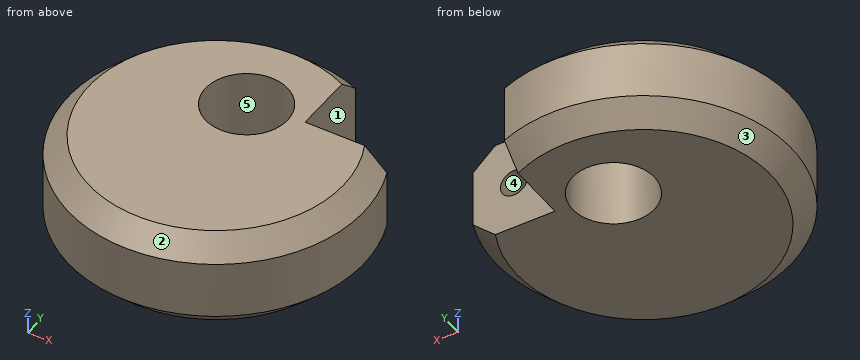
from build123d import *

# Parameters (mm, degrees)
SKETCH1_R             = 18
BOSS_EXTRUDE1_DEPTH   = 12
CUT_EXTRUDE4_DEPTH    = 17
SKETCH1_5_R           = 5
CUT_EXTRUDE5_DEPTH    = 22
M4_TAPPED_HOLE1_D     = 3.3
M4_TAPPED_HOLE1_DEPTH = 14
M4_TAPPED_HOLE1_TIP   = 0.991420021
CHAMFER1_SIZE         = 2.5
CHAMFER2_SIZE         = 2.5


with BuildPart() as part:
    # Sketch1 → Boss-Extrude1 (new body)
    with BuildSketch(Plane.XY):
        Circle(SKETCH1_R)
    extrude(amount=-BOSS_EXTRUDE1_DEPTH)

    # Sketch1<4> → Cut-Extrude4 (cut)
    with BuildSketch(Plane.XY):
        with BuildLine():
            Line((16.704699911, 6.704699911), (6.704699911, 6.704699911))
            Line((6.704699911, 6.704699911), (6.704699911, 16.704699911))
            ThreePointArc((6.704699911, 16.704699911), (12.727922061, 12.727922061), (16.704699911, 6.704699911))
        make_face()
    extrude(amount=-CUT_EXTRUDE4_DEPTH, mode=Mode.SUBTRACT)

    # Sketch1<5> → Cut-Extrude5 (cut)
    with BuildSketch(Plane.XY):
        with Locations((0, 6)):
            Circle(SKETCH1_5_R)
    extrude(amount=-CUT_EXTRUDE5_DEPTH, mode=Mode.SUBTRACT)

    # M4 Tapped Hole1
    with Locations(Plane(origin=(0, 6.704699911, 0), x_dir=(1, 0, 0), z_dir=(0, 1, 0))):
        with Locations((11.704699911, 6)):
            Hole(M4_TAPPED_HOLE1_D / 2, depth=M4_TAPPED_HOLE1_DEPTH)
            with Locations((0, 0, -(M4_TAPPED_HOLE1_DEPTH + M4_TAPPED_HOLE1_TIP / 2))):  # 118° drill point
                Cone(0, M4_TAPPED_HOLE1_D / 2, M4_TAPPED_HOLE1_TIP, mode=Mode.SUBTRACT)

    # Chamfer1
    chamfer1_edges = [part.edges().sort_by_distance(p)[0] for p in [
        (-12.727922061, -12.727922061, 0),
    ]]
    chamfer(chamfer1_edges, length=CHAMFER1_SIZE)

    # Chamfer2
    chamfer2_edges = [part.edges().sort_by_distance(p)[0] for p in [
        (-12.727922061, -12.727922061, -12),
    ]]
    chamfer(chamfer2_edges, length=CHAMFER2_SIZE)


solid = part.part
CAD build for the part. Positions are in the model's coordinates, mm. Face numbers are marked on the shaded views. A direction names the side the tool comes from. Round coordinates to 2 decimals unless told otherwise and drop trailing zeros. Write each loop counter-clockwise with the first axis right and the second up, starting at its lowest first coordinate (ties: lowest second). Pieces come first, ordered by that corner, then holes.
(1) Slice it at C-C, the plane y = 6. Count the separate pieces of the cut face and the enclosed holes in it, and give its area (3 significant figures).
(2) Mould opens along Z. For the marked faces 3, 4 and 5 say: pulls with the +Z half, pulls with the -Z half, needs draft (parallel to the pull), parting line crosses it, or undercut.
(3) 3-axis set-ups, long thin cutter, end or side, ignore diameter. For the marked faces 1 and 2: which of +Z, -Z, +X, -X, +Y, -Y reach the whole face in a straight line?
(4) Slice it at D-D, the plane z = -1. Write the cut outline in (x, y), and give its area (3 significant figures).
(5) Probe line 1 along X through (y, z) = (3, -6); line 2 along X through (y, z) = (1.75, -6); line 3 along Y through (x, z) = (-4.5, -8.5). List the from-to ranges inside material, lowest first.
(6) Drop flat-ended pins along their axis: P1, Ø5, axis at x = -7.5, z = -9, coming from the +Y side; P2, Ø9, axis at x = 0, y = 6, coming from the -Z side; P3, Ø5, axis at y = 13, z = -5, coming from the +X side; P4, Ø2, axis at x = 11.7, z = -6, coming from the -Y side. Give the stop position or say it passes through.
(7) Slice it at B-B, the plane z = -9. Write the cut outline in (x, y).
(8) Slice it at A-A, the plane y = 0. Write the cut outline in (x, z).
From the geometry:
1. separate pieces: 2
1. enclosed holes: 1
1. area: 265 mm2
2. face 3: pulls with the -Z half
2. face 4: undercut
2. face 5: needs draft
3. face 1: +Z, -Z, +X, +Y
3. face 2: +Z
4. outline: (6.7, 6.7) - (6.7, 15.08) arc R16.5 ccw (long way) to (15.08, 6.7) - close; hole circle Ø10 at (0, 6)
4. area: 733 mm2
5. line 1: x = -17.75 to -4, 4 to 10.05, 13.35 to 17.75
5. line 2: x = -17.91 to -2.63, 2.63 to 10.05, 13.35 to 17.91
5. line 3: y = -17.43 to 3.82, 8.18 to 17.43
6. P1: stops at y = 17.29
6. P2: passes through
6. P3: stops at x = 6.7
6. P4: stops at y = -14.47
7. outline: (6.7, 6.7) - (6.7, 16.7) arc R18 ccw (long way) to (16.7, 6.7) - close; hole circle Ø10 at (0, 6)
8. outline: (-18, -9.5) - (-15.5, -12) - (15.5, -12) - (18, -9.5) - (18, -2.5) - (15.5, 0) - (-15.5, 0) - (-18, -2.5) - close; hole circle Ø3.3 at (11.7, -6)
